from build123d import *

# Parameters (mm, degrees)
BOX_W           = 27
BOX_H           = 12
BOX_DEPTH       = 48
SKETCH_W        = 23.5
SKETCH_H        = 20
POCKET_DEPTH    = 10
SKETCH002_R     = 1
POCKET001_DEPTH = 28.001
SKETCH003_R     = 3
POCKET002_DEPTH = 26.5
SKETCH004_R     = 2.4
POCKET003_DEPTH = 2.001
POCKET004_DEPTH = 2.001
PAD_DEPTH       = 2
FILLET_R        = 1
FILLET001_R     = 0.8


with BuildPart() as part:
    # Box → Box (new body)
    with BuildSketch(Plane.XY):
        with Locations((13.5, 6)):
            Rectangle(BOX_W, BOX_H)
    extrude(amount=BOX_DEPTH)

    # Sketch (on Face3 of BaseFeature) → Pocket (cut)
    with BuildSketch(Plane.XZ):
        with Locations((13.5, 10)):
            Rectangle(SKETCH_W, SKETCH_H)
    extrude(amount=-POCKET_DEPTH, mode=Mode.SUBTRACT)

    # Sketch002 (on Face7 of Pocket) → Pocket001 (cut, through all)
    with BuildSketch(Plane(origin=(0, 0, 20), x_dir=(1, 0, 0), z_dir=(0, 0, -1))):
        with Locations((13.5, -5)):
            Circle(SKETCH002_R)
    extrude(amount=-POCKET001_DEPTH, mode=Mode.SUBTRACT)

    # Sketch003 (on Face7 of Pocket001) → Pocket002 (cut)
    with BuildSketch(Plane(origin=(0, 0, 20), x_dir=(1, 0, 0), z_dir=(0, 0, -1))):
        with Locations((13.5, -5)):
            Circle(SKETCH003_R)
    extrude(amount=-POCKET002_DEPTH, mode=Mode.SUBTRACT)

    # Sketch004 (on Face11 of Pocket002) → Pocket003 (cut, through all)
    with BuildSketch(Plane.XZ.offset(-10)):
        with Locations((4.75, 8.5)):
            Circle(SKETCH004_R)
        with Locations((22.25, 8.5)):
            Circle(SKETCH004_R)
    extrude(amount=-POCKET003_DEPTH, mode=Mode.SUBTRACT)

    # Sketch005 (on Face13 of Pocket003) → Pocket004 (cut, through all)
    with BuildSketch(Plane.XZ.offset(-10)):
        with BuildLine():
            ThreePointArc((16, 0), (13.5, 2.5), (11, 0))
            Line((11, 0), (16, 0))
        make_face()
    extrude(amount=-POCKET004_DEPTH, mode=Mode.SUBTRACT)

    # Sketch006 (on Face3 of Pocket004) → Pad (join)
    with BuildSketch(Plane.XY.offset(48)):
        Polygon((3.4, 9.497498), (1.402502, 9.397498), (1.502502, 7.4), (3.5, 7.5), align=None)
        Polygon((1.502502, 2.6), (3.5, 2.5), (3.4, 0.502502), (1.402502, 0.602502), align=None)
        Polygon((23.5, 2.5), (25.497498, 2.6), (25.597498, 0.602502), (23.6, 0.502502), align=None)
        Polygon((23.6, 9.497498), (25.597498, 9.397498), (25.497498, 7.4), (23.5, 7.5), align=None)
    extrude(amount=PAD_DEPTH)

    # Fillet
    fillet_edges = [part.edges().sort_by_distance(p)[0] for p in [
        (27, 6, 48),
        (27, 12, 24),
        (13.5, 12, 48),
        (0, 12, 24),
        (0, 6, 48),
    ]]
    fillet(fillet_edges, radius=FILLET_R)

    # Fillet001
    fillet001_edges = [part.edges().sort_by_distance(p)[0] for p in [
        (2.401251, 9.447498, 50),
        (2.401251, 0.552502, 50),
        (24.598749, 9.447498, 50),
        (24.598749, 0.552502, 50),
    ]]
    fillet(fillet001_edges, radius=FILLET001_R)


solid = part.part
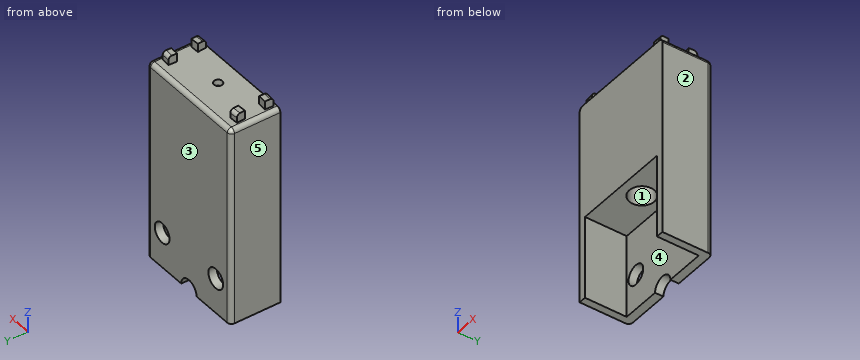
Geometry: final body of the model. Coordinates: model frame, mm. Face numbers are marked on the shaded views. A direction names the side the tool comes from. Give positions to 0.01 mm unless a question says otherwise; leave off trailing zeros. Write each loop counter-clockwise with the first axis right and the second up, starting at its lowest first coordinate (ties: lowest second). Pieces come first, ordered by that corner, then holes.
(1) Ray query, line 1 (X direction, y = 8, z = 17.5); line 2 (X direction, y = 5, z = 24.5); line 3 (Z direction, x = 22.25, y = 10.4). Return the intervals inside material, ascending.
(2) Cut plane C-C, the plane y = 5. Return loops of the section in (x, z).
(3) First-contact query: P1, Ø7.5, axis at x = 4.75, z = 8.5, coming from the +Y side; P2, Ø1, axis at x = 13.5, y = 3, coming from the +Z side; P3, Ø6, axis at x = 9.5, z = 12, coming from the -Y side; P4, Ø6.5, axis at x = 14, y = 5.5, coming from the -Z side. Flat tips, straight axial feed; report the tip coordinate or a pass-through.
(4) Cut plane D-D, the plane z = 8.5. Return loops of the section in (x, y).
(5) Cut plane B-B, the plane z = 43.5. Return loops of the section in (x, y), then the cut area to 3 significant figures.
(6) Access query for the marked faces 4 and 5. Directions: +Z, -Z, +X, -X, +Y, -Y. A direction counts if a zero-diameter tool reaches every point of the face in a straight line with its end or side. Return the directions, or none.
(7) Mould query, pull axis X, two halves, no side actions, for the marked faces 1, 2 and 3. Classes: released by +X, released by -X, zero draft, split by the parting line, or undercut.
(8) Cut plane A-A, the plane x = 4.75. Return loops of the section in (y, z), then the cut area to 3 significant figures.
Values follow:
1. line 1: x = 0 to 1.75, 25.25 to 27
1. line 2: x = 0 to 10.5, 16.5 to 27
1. line 3: z = 0 to 6.1, 10.9 to 48
2. outline: (0, 0) - (1.75, 0) - (1.75, 20) - (10.5, 20) - (10.5, 46.5) - (12.5, 46.5) - (12.5, 48) - (1, 48) arc R1 ccw to (0, 47) - close; (14.5, 46.5) - (16.5, 46.5) - (16.5, 20) - (25.25, 20) - (25.25, 0) - (27, 0) - (27, 47) arc R1 ccw to (26, 48) - (14.5, 48) - close
3. P1: stops at y = 12
3. P2: stops at z = 48
3. P3: stops at y = 10
3. P4: stops at z = 20
4. outline: (0, 0) - (1.75, 0) - (1.75, 10) - (2.35, 10) - (2.35, 12) - (1, 12) arc R1 ccw to (0, 11) - close; (7.15, 10) - (19.85, 10) - (19.85, 12) - (7.15, 12) - close; (24.65, 10) - (25.25, 10) - (25.25, 0) - (27, 0) - (27, 11) arc R1 ccw to (26, 12) - (24.65, 12) - close
5. outline: (0, 0) - (27, 0) - (27, 11) arc R1 ccw to (26, 12) - (1, 12) arc R1 ccw to (0, 11) - close; hole circle Ø6 at (13.5, 5)
5. area: 295 mm2
6. face 4: -Z, -Y
6. face 5: +Z, -Z, -X, +Y, -Y
7. face 1: undercut
7. face 2: released by +X
7. face 3: zero draft
8. outline: (0, 20) - (10, 20) - (10, 10.9) - (12, 10.9) - (12, 47) arc R1 ccw to (11, 48) - (0, 48) - close; (10, 0) - (12, 0) - (12, 6.1) - (10, 6.1) - close
8. area: 366 mm2
